Design review of the part built by this model. Coordinates are the model's own, in mm. A direction names the side the tool comes from. Give positions to 0.01 mm unless a question says otherwise; leave off trailing zeros. Write each loop counter-clockwise with the first axis right and the second up, starting at its lowest first coordinate (ties: lowest second). Pieces come first, ordered by that corner, then holes.
```python
from build123d import *

# Parameters (mm, degrees)
RESSALTO_EXTRUS_O1_DEPTH = 1.4
ESBO_O2_R                = 3.45
RESSALTO_EXTRUS_O2_DEPTH = 2.4
FURO1_D                  = 1.2
PADR_O_LINEAR1_COUNT     = 6
PADR_O_LINEAR1_PITCH     = 2
RESSALTO_EXTRUS_O3_DEPTH = 1.4
FURO2_D                  = 1.2
PADR_O_LINEAR2_COUNT     = 7
PADR_O_LINEAR2_PITCH     = 2
RESSALTO_EXTRUS_O4_DEPTH = 1.4
FURO3_D                  = 1.2
PADR_O_LINEAR3_COUNT     = 2
PADR_O_LINEAR3_PITCH     = 2
PADR_OCIRCULAR1_COUNT    = 2
PADR_OCIRCULAR1_COPY_1_D = 1.2
FURO4_D                  = 5
FURO4_DEPTH              = 2
FURO5_D                  = 4.6
FURO5_DEPTH              = 1
FURO6_D                  = 2.1


with BuildPart() as part:
    # Esboço1 → Ressalto-extrusão1 (new body)
    with BuildSketch(Plane(origin=(0, 0, 0), x_dir=(1, 0, 0), z_dir=(0, 1, 0))):
        with BuildLine():
            Line((-14.159121967, 1.99702088), (-2.209072203, 2.65))
            ThreePointArc((-2.209072203, 2.65), (3.45, 0), (-2.209072203, -2.65))
            Line((-2.209072203, -2.65), (-14.159121967, -1.99702088))
            ThreePointArc((-14.159121967, -1.99702088), (-16.05, 0), (-14.159121967, 1.99702088))
        make_face()
    extrude(amount=-RESSALTO_EXTRUS_O1_DEPTH)

    # Esboço2 → Ressalto-extrusão2 (add)
    with BuildSketch(Plane.XZ.offset(1.4)):
        with Locations(Location((0, 0, 0), (0, 0, 90))):
            Circle(ESBO_O2_R)
    extrude(amount=RESSALTO_EXTRUS_O2_DEPTH)

    # Furo1 (through all)
    with Locations(Plane(origin=(0, 0, 0), x_dir=(1, 0, 0), z_dir=(0, 1, 0))):
        with Locations((-14.45, 0)):
            furo1 = Hole(FURO1_D / 2)

    # Padrão linear1: Furo1 ×6
    with Locations(*[(i * PADR_O_LINEAR1_PITCH, 0, 0) for i in range(1, PADR_O_LINEAR1_COUNT)]):
        add(furo1, mode=Mode.SUBTRACT)

    # Esboço12 → Ressalto-extrusão3 (add)
    with BuildSketch(Plane(origin=(0, 0, 0), x_dir=(1, 0, 0), z_dir=(0, 1, 0))):
        with BuildLine():
            Line((0.304103343, 3.436571134), (16.626291793, 1.99221515))
            ThreePointArc((16.626291793, 1.99221515), (18.45, 0), (16.626291793, -1.99221515))
            Line((16.626291793, -1.99221515), (0.304103343, -3.436571134))
            ThreePointArc((0.304103343, -3.436571134), (3.45, 0), (0.304103343, 3.436571134))
        make_face()
    extrude(amount=-RESSALTO_EXTRUS_O3_DEPTH)

    # Furo2 (through all)
    with Locations(Plane(origin=(0, 0, 0), x_dir=(1, 0, 0), z_dir=(0, 1, 0))):
        with Locations((16.85, 0)):
            furo2 = Hole(FURO2_D / 2)

    # Padrão linear2: Furo2 ×7
    with Locations(*[(-i * PADR_O_LINEAR2_PITCH, 0, 0) for i in range(1, PADR_O_LINEAR2_COUNT)]):
        add(furo2, mode=Mode.SUBTRACT)

    # Esboço16 → Ressalto-extrusão4 (add)
    with BuildSketch(Plane(origin=(0, 0, 0), x_dir=(1, 0, 0), z_dir=(0, 1, 0))):
        with BuildLine():
            Line((-1.9, -6.45), (-1.9, 6.45))
            ThreePointArc((-1.9, 6.45), (0, 8.35), (1.9, 6.45))
            Line((1.9, 6.45), (1.9, -6.45))
            ThreePointArc((1.9, -6.45), (0, -8.35), (-1.9, -6.45))
        make_face()
    extrude(amount=-RESSALTO_EXTRUS_O4_DEPTH)

    # Furo3 (through all)
    with Locations(Plane(origin=(0, 0, 0), x_dir=(1, 0, 0), z_dir=(0, 1, 0))):
        with Locations((0, -6.45)):
            furo3 = Hole(FURO3_D / 2)

    # Padrão linear3: Furo3 ×2
    with Locations(*[(0, 0, -i * PADR_O_LINEAR3_PITCH) for i in range(1, PADR_O_LINEAR3_COUNT)]):
        add(furo3, mode=Mode.SUBTRACT)

    # PadrãoCircular1: Furo3 ×2 about axis
    padr_ocircular1_axis = Axis((0, 0, 0), (0, 1, 0))
    for i in range(1, PADR_OCIRCULAR1_COUNT):
        add(furo3.rotate(padr_ocircular1_axis, i * 360 / PADR_OCIRCULAR1_COUNT), mode=Mode.SUBTRACT)

    # PadrãoCircular1 copy 1 (through all)
    with Locations(Plane(origin=(0, 0, 2), x_dir=(-1, 0, 0), z_dir=(0, 1, 0))):
        with Locations((0, -6.45)):
            Hole(PADR_OCIRCULAR1_COPY_1_D / 2)

    # Furo4
    with Locations(Plane(origin=(0, -3.8, 0), x_dir=(-1, 0, 0), z_dir=(0, -1, 0))):
        with Locations((0, 0)):
            Hole(FURO4_D / 2, depth=FURO4_DEPTH)

    # Furo5
    with Locations(Plane(origin=(0, 0, 0), x_dir=(1, 0, 0), z_dir=(0, 1, 0))):
        with Locations((0, 0)):
            Hole(FURO5_D / 2, depth=FURO5_DEPTH)

    # Furo6 (through all)
    with Locations(Plane(origin=(0, 0, 0), x_dir=(1, 0, 0), z_dir=(0, 1, 0))):
        with Locations((0, 0)):
            Hole(FURO6_D / 2)


solid = part.part
```
(1) Tool access review of faces 1 (the face through (1.9, -1, -5)), 2 (the face through (-1.9, -1, -5)), 3 (the face through (1, -1.8, 1)): name each direction out of +Z, -Z, +X, -X, +Y, -Y from which nothing blocks a thin tool from reaching the whole face with its end or side.
Resolved:
face 1: -Z, +X, +Y, -Y
face 2: -Z, -X, +Y, -Y
face 3: -Y
(2) Consider section B-B, the plane x = 8.85. Give the boundary of the cut face in (y, z).
Resolved:
outline: (-1.4, -2.68) - (0, -2.68) - (0, -0.6) - (-1.4, -0.6) - close; (-1.4, 0.6) - (0, 0.6) - (0, 2.68) - (-1.4, 2.68) - close
(3) Consider section A-A, the plane x = -12.45. Give the boundary of the cut face in (y, z), then the cut area to 3 significant figures.
Resolved:
outline: (-1.4, -2.09) - (0, -2.09) - (0, -0.6) - (-1.4, -0.6) - close; (-1.4, 0.6) - (0, 0.6) - (0, 2.09) - (-1.4, 2.09) - close
area: 4.17 mm2
(4) Clearance check with flat-ended pins moving along their axes: P1, Ø1.5, axis at y = -0.5, z = 5.5, coming from the -X side; P2, Ø2.5, axis at x = 0, z = -1, coming from the -Y side; P3, Ø1.4, axis at x = 0.5, z = -1, coming from the +Y side. State where each tip first meets the part, or that it passes through.
Resolved:
P1: stops at x = -1.9
P2: stops at y = -1.8
P3: stops at y = -1
(5) To check wall thickness, follow L1, parallel to Z at x = 0, y = -0.7; L2, parallel to X at y = -0.55, z = 6.45; L3, parallel to Y at x = 7, z = -2. State the ranges of each line that lie inside material, in increasing order.
Resolved:
L1: z = -8.35 to -7.05, -5.85 to -5.05, -3.85 to -2.3, 2.3 to 3.85, 5.05 to 5.85, 7.05 to 8.35
L2: x = -1.9 to -0.6, 0.6 to 1.9
L3: y = -1.4 to 0
(6) Mouldability with a two-part tool opening along Z and no side actions: class faces 4 (the face through (-16.05, -0.69, 0.04)), 5 (the face through (0.04, -0.69, 8.35)), 6 (the face through (1.825, -0.507, 1.4)) as pulls with the +Z half, pulls with the -Z half, needs draft (parallel to the pull), parting line crosses it, or undercut.
Resolved:
face 4: parting line crosses it
face 5: pulls with the +Z half
face 6: undercut
